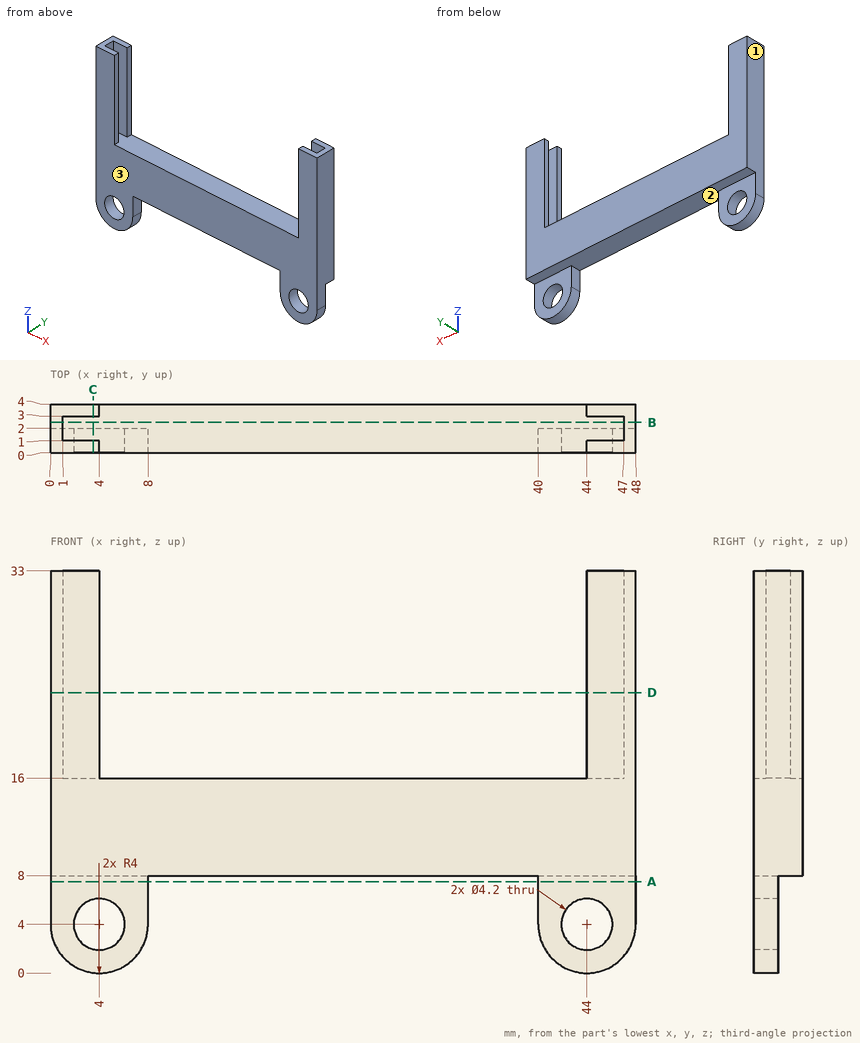
Drawing for the job (mm, zero at the part's lowest x, y, z). Round coordinates to 2 decimals unless told otherwise and drop trailing zeros. Loops run counter-clockwise (first coordinate to the right, second up) from the corner with the lowest first, then second, coordinate; pieces in that order, holes last.
1. Wall check: probe 1 along X at (y, z) = (1.35, 28.5); probe 2 along X at (y, z) = (3.55, 19); probe 3 along Z at (x, y) = (9, 2.2). Give the ranges that are in metal, low to high.
Check values:
probe 1: x = 0 to 1, 47 to 48
probe 2: x = 0 to 4, 44 to 48
probe 3: z = 8 to 16
2. Band-saw the part on D-D, the plane z = 23. List the corners of the cut face in (x, y).
Check values:
outline: (0, 0) - (4, 0) - (4, 1) - (1, 1) - (1, 3) - (4, 3) - (4, 4) - (0, 4) - close; (44, 0) - (48, 0) - (48, 4) - (44, 4) - (44, 3) - (47, 3) - (47, 1) - (44, 1) - close
3. Band-saw the part on C-C, the plane x = 3.5. List the corners of the cut face in (y, z).
Check values:
outline: (0, 0.03) - (2, 0.03) - (2, 1.96) - (0, 1.96) - close; (0, 6.04) - (2, 6.04) - (2, 8) - (4, 8) - (4, 33) - (3, 33) - (3, 16) - (1, 16) - (1, 33) - (0, 33) - close
4. Mould opens along X. For the marked faces 1, 2 and 3 say: +X half, -X half, draft (parallel to the pull), parting line (faces both ways), or undercut.
Check values:
face 1: -X half
face 2: undercut
face 3: draft
5. Band-saw the part on A-A, the plane z = 7.5. List the corners of the cut face in (x, y).
Check values:
outline: (0, 0) - (8, 0) - (8, 2) - (0, 2) - close; (40, 0) - (48, 0) - (48, 2) - (40, 2) - close
6. Drop flat-ended pins along their axis: P1, Ø4, axis at x = 45.5, z = 3, coming from the +Y side; P2, Ø1.2, axis at x = 27, y = 2.5, coming from the -Z side; P3, Ø2, axis at x = 36.5, y = 0.5, coming from the +Z side. Give the stop position or say it passes through.
Check values:
P1: stops at y = 2
P2: stops at z = 8
P3: stops at z = 16
7. Band-saw the part on B-B, the plane y = 2.5. List the corners of the cut face in (x, z).
Check values:
outline: (0, 8) - (48, 8) - (48, 33) - (47, 33) - (47, 16) - (1, 16) - (1, 33) - (0, 33) - close
